Geometry: final body of the model. Coordinates: model frame, mm. Face numbers are marked on the shaded views. A direction names the side the tool comes from. Give positions to 0.01 mm unless a question says otherwise; leave off trailing zeros. Write each loop counter-clockwise with the first axis right and the second up, starting at its lowest first coordinate (ties: lowest second). Pieces come first, ordered by that corner, then holes. Notation, with made-up numbers: M -34.5,-27.5 L 12.5,-27.5 A32 ccw 12.5,3.5 Z; hole C 82.5,46.5 d2. An arc over 180 degrees is marked long. Answer as a JSON object with one key per item and string values.
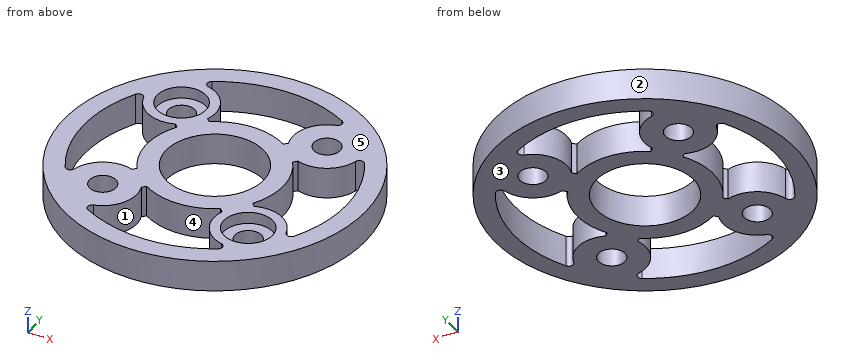
from build123d import *

# Parameters (mm, degrees)
F0_R            = 24.51608
F0_R_2          = 2.15265
F0_R_3          = 7.9375
F1_DEPTH        = 5.08
F3_DEPTH        = 5.08
F3_COPIES_COUNT = 4
F4_R            = 0.762
F5_R            = 3.96875
F6_DEPTH        = 1.905


# Not quite as in the source:
# - a pattern or mirror of a feature is missing from the dataset's text; its kind, count and spacing are read off the source's solid


with BuildPart() as f1:
    # F0 (on Top) → F1 (new body)
    with BuildSketch(Plane.XY):
        Circle(F0_R)
        with Locations((-11.7865906, -11.7865906)):
            Circle(F0_R_2, mode=Mode.SUBTRACT)
        with Locations((11.7865906, -11.7865906)):
            Circle(F0_R_2, mode=Mode.SUBTRACT)
        with Locations((-11.7865906, 11.7865906)):
            Circle(F0_R_2, mode=Mode.SUBTRACT)
        Circle(F0_R_3, mode=Mode.SUBTRACT)
        with Locations((11.7865906, 11.7865906)):
            Circle(F0_R_2, mode=Mode.SUBTRACT)
    extrude(amount=F1_DEPTH)

    # F2 (on face) → F3 (cut, through all)
    with BuildSketch(Plane.XY.offset(5.08)):
        with BuildLine():
            ThreePointArc((-12.5005198818, 17.2967828873), (-7.4612395718, 15.2741760893), (-6.553034663, 9.9206307084))
            Line((-6.553034663, 9.9206307084), (-5.9913991959, 9.3589952413))
            ThreePointArc((-5.9913991959, 9.3589952413), (0, 11.1125), (5.9913991959, 9.3589952413))
            Line((5.9913991959, 9.3589952413), (6.553034663, 9.9206307084))
            ThreePointArc((6.553034663, 9.9206307084), (7.4612395718, 15.2741760893), (12.5005198818, 17.2967828873))
            ThreePointArc((12.5005198818, 17.2967828873), (0, 21.34108), (-12.5005198818, 17.2967828873))
        make_face()
    f3 = extrude(amount=-F3_DEPTH, mode=Mode.SUBTRACT)

    # F3_copies: F3 ×4 about axis
    f3_copies_axis = Axis((0, 0, 0), (0, 0, 1))
    for i in range(1, F3_COPIES_COUNT):
        add(f3.rotate(f3_copies_axis, i * 360 / F3_COPIES_COUNT), mode=Mode.SUBTRACT)

    # F4
    f4_edges = [f1.edges().sort_by_distance(p)[0] for p in [
        (-12.50052, 17.296783, 2.54),
        (12.50052, 17.296783, 2.54),
        (-17.296783, -12.50052, 2.54),
        (-17.296783, 12.50052, 2.54),
        (12.50052, -17.296783, 2.54),
        (-12.50052, -17.296783, 2.54),
        (17.296783, 12.50052, 2.54),
        (17.296783, -12.50052, 2.54),
    ]]
    fillet(f4_edges, radius=F4_R)

    # F5 (on face) → F6 (cut)
    with BuildSketch(Plane.XY.offset(5.08)):
        with Locations((-11.7865906, 11.7865906)):
            Circle(F5_R)
        with Locations((11.7865906, -11.7865906)):
            Circle(F5_R)
    extrude(amount=-F6_DEPTH, mode=Mode.SUBTRACT)


solid = f1.part
1) Contact query for flat-ended pins moving along their axis: P1, Ø5, axis at x = 11.79, y = -11.79, coming from the +Z side (3 decimals); P2, Ø2, axis at y = 12, z = 2, coming from the +X side; P3, Ø1.5, axis at y = -8, z = 3, coming from the +X side; P4, Ø1.5, axis at x = -9.5, y = 10, coming from the -Z side. Output: stop coordinate, or through.
Geometry check:
{"P1": "stops at z = 3.175", "P2": "stops at x = 21.91", "P3": "stops at x = 23.42", "P4": "stops at z = 0"}
2) Cut plane A-A on y = 0. Return loops of the section in (x, z).
Geometry check:
{"outline": "M -24.52,0 L -21.34,0 L -21.34,5.08 L -24.52,5.08 Z; M -11.11,0 L -7.94,0 L -7.94,5.08 L -11.11,5.08 Z; M 7.94,0 L 11.11,0 L 11.11,5.08 L 7.94,5.08 Z; M 21.34,0 L 24.52,0 L 24.52,5.08 L 21.34,5.08 Z"}
3) Set-up query: the marked faces 4 and 5. Return all of +Z, -Z, +X, -X, +Y, -Y with unobstructed straight access to the full face (end or side cutting, diameter ignored); none if empty.
Geometry check:
{"face 4": "+Z, -Z", "face 5": "+Z, +X, -X, +Y, -Y"}
4) Line query: line 1 (Y direction, x = -11.5, z = 2.45); line 2 (X direction, y = 2.5, z = 3.05); line 3 (X direction, y = -14.5, z = 3.9). Output: solid intervals per line, ascending. Write a range as from..to.
Geometry check:
{"line 1": "y = -21.65..-13.92, -9.65..-6.24, 6.24..9.65, 13.92..21.65", "line 2": "x = -24.39..-21.19, -10.83..-7.53, 7.53..10.83, 21.19..24.39", "line 3": "x = -19.77..-6.94, 6.94..8.89, 14.68..19.77"}
5) Cut plane D-D on z = 1.05. Give the number of separate pieces and of enclosed holes in the cut face, and give its area (3 significant figures).
Geometry check:
{"separate pieces": "1", "enclosed holes": "9", "area": "973 mm2"}
6) Pull-direction query (Y, two-part tool) for the marked faces 1, 2 and 3; classes: pulls with the +Y half, pulls with the -Y half, needs draft (parallel to the pull), parting line crosses it, or undercut.
Geometry check:
{"face 1": "undercut", "face 2": "parting line crosses it", "face 3": "needs draft"}
7) Cut plane C-C on x = -19.5. Return loops of the section in (y, z).
Geometry check:
{"outline": "M -14.86,0 L -8.67,0 L -8.67,5.08 L -14.86,5.08 Z; M 8.67,0 L 14.86,0 L 14.86,5.08 L 8.67,5.08 Z"}
